Here's how the part is built. I have some questions about the finished solid (model axes, mm). A direction names the side the tool comes from. Coordinates: 2 decimals unless noted, no trailing zeros. Loops run counter-clockwise (first coordinate to the right, second up) from the corner with the lowest first, then second, coordinate; pieces in that order, holes last. Notation, with made-up numbers: (46.25, -16) - (99.25, -16) arc R16 cw to (99.25, -8) - close; hole circle Ø2 at (80.25, -29). An arc over 180 degrees is marked (long way). Use a Markdown table: item, result.
```python
from build123d import *

# Parameters (mm, degrees)
F1_DEPTH = 914.4
F2_W     = 762
F2_H     = 762
F3_DEPTH = 3.175
F4_R     = 12.7
F6_DEPTH = 228.6


with BuildPart() as f1:
    # F0 (on Top) → F1 (new body)
    with BuildSketch(Plane.XY):
        with BuildLine():
            Line((-19.3675, -30.95625), (0, -30.95625))
            Line((0, -30.95625), (19.3675, -30.95625))
            ThreePointArc((19.3675, -30.95625), (20.265526, -30.584276), (20.6375, -29.68625))
            Line((20.6375, -29.68625), (20.6375, 29.68625))
            ThreePointArc((20.6375, 29.68625), (20.265526, 30.584276), (19.3675, 30.95625))
            Line((19.3675, 30.95625), (15.5575, 30.95625))
            ThreePointArc((15.5575, 30.95625), (14.659474, 30.584276), (14.2875, 29.68625))
            Line((14.2875, 29.68625), (14.2875, 24.60625))
            Line((14.2875, 24.60625), (15.29505, 24.60625))
            Line((15.29505, 24.60625), (15.29505, 29.68625))
            ThreePointArc((15.29505, 29.68625), (15.37192, 29.87183), (15.5575, 29.9487))
            Line((15.5575, 29.9487), (19.3675, 29.9487))
            ThreePointArc((19.3675, 29.9487), (19.55308, 29.87183), (19.62995, 29.68625))
            Line((19.62995, 29.68625), (19.62995, -29.68625))
            ThreePointArc((19.62995, -29.68625), (19.55308, -29.87183), (19.3675, -29.9487))
            Line((19.3675, -29.9487), (0, -29.9487))
            Line((0, -29.9487), (-19.3675, -29.9487))
            ThreePointArc((-19.3675, -29.9487), (-19.55308, -29.87183), (-19.62995, -29.68625))
            Line((-19.62995, -29.68625), (-19.62995, 29.68625))
            ThreePointArc((-19.62995, 29.68625), (-19.55308, 29.87183), (-19.3675, 29.9487))
            Line((-19.3675, 29.9487), (-15.5575, 29.9487))
            ThreePointArc((-15.5575, 29.9487), (-15.37192, 29.87183), (-15.29505, 29.68625))
            Line((-15.29505, 29.68625), (-15.29505, 24.60625))
            Line((-15.29505, 24.60625), (-14.2875, 24.60625))
            Line((-14.2875, 24.60625), (-14.2875, 29.68625))
            ThreePointArc((-14.2875, 29.68625), (-14.659474, 30.584276), (-15.5575, 30.95625))
            Line((-15.5575, 30.95625), (-19.3675, 30.95625))
            ThreePointArc((-19.3675, 30.95625), (-20.265526, 30.584276), (-20.6375, 29.68625))
            Line((-20.6375, 29.68625), (-20.6375, -29.68625))
            ThreePointArc((-20.6375, -29.68625), (-20.265526, -30.584276), (-19.3675, -30.95625))
        make_face()
    extrude(amount=F1_DEPTH)

    # F2 (on Top) → F3 (join)
    with BuildSketch(Plane.XY):
        Rectangle(F2_W, F2_H)
    extrude(amount=-F3_DEPTH)

    # F4
    f4_edges = [f1.edges().sort_by_distance(p)[0] for p in [
        (381, -381, -1.5875),
        (381, 381, -1.5875),
        (-381, 381, -1.5875),
        (-381, -381, -1.5875),
    ]]
    fillet(f4_edges, radius=F4_R)

    # F5 (on Right) → F6 (join, symmetric)
    with BuildSketch(Plane.YZ):
        with BuildLine():
            Line((-29.9487, 915.67), (-29.9487, 954.405))
            ThreePointArc((-29.9487, 954.405), (-29.87183, 954.59058), (-29.68625, 954.66745))
            Line((-29.68625, 954.66745), (29.68625, 954.66745))
            ThreePointArc((29.68625, 954.66745), (29.87183, 954.59058), (29.9487, 954.405))
            Line((29.9487, 954.405), (29.9487, 950.595))
            ThreePointArc((29.9487, 950.595), (29.87183, 950.40942), (29.68625, 950.33255))
            Line((29.68625, 950.33255), (24.60625, 950.33255))
            Line((24.60625, 950.33255), (24.60625, 949.325))
            Line((24.60625, 949.325), (29.68625, 949.325))
            ThreePointArc((29.68625, 949.325), (30.584276, 949.696974), (30.95625, 950.595))
            Line((30.95625, 950.595), (30.95625, 954.405))
            ThreePointArc((30.95625, 954.405), (30.584276, 955.303026), (29.68625, 955.675))
            Line((29.68625, 955.675), (-29.68625, 955.675))
            ThreePointArc((-29.68625, 955.675), (-30.584276, 955.303026), (-30.95625, 954.405))
            Line((-30.95625, 954.405), (-30.95625, 935.0375))
            Line((-30.95625, 935.0375), (-30.95625, 915.67))
            ThreePointArc((-30.95625, 915.67), (-30.584276, 914.771974), (-29.68625, 914.4))
            Line((-29.68625, 914.4), (29.68625, 914.4))
            ThreePointArc((29.68625, 914.4), (30.584276, 914.771974), (30.95625, 915.67))
            Line((30.95625, 915.67), (30.95625, 919.48))
            ThreePointArc((30.95625, 919.48), (30.584276, 920.378026), (29.68625, 920.75))
            Line((29.68625, 920.75), (24.60625, 920.75))
            Line((24.60625, 920.75), (24.60625, 919.74245))
            Line((24.60625, 919.74245), (29.68625, 919.74245))
            ThreePointArc((29.68625, 919.74245), (29.87183, 919.66558), (29.9487, 919.48))
            Line((29.9487, 919.48), (29.9487, 915.67))
            ThreePointArc((29.9487, 915.67), (29.87183, 915.48442), (29.68625, 915.40755))
            Line((29.68625, 915.40755), (-29.68625, 915.40755))
            ThreePointArc((-29.68625, 915.40755), (-29.87183, 915.48442), (-29.9487, 915.67))
        make_face()
    extrude(amount=F6_DEPTH, both=True)


solid = f1.part
```
Q1. Will these pins go through, and if not, where does the flat tip stop? P1, Ø4, axis at x = -38, z = 953, coming from the +Y side; P2, Ø1.5, axis at x = -196.5, y = -188.5, coming from the +Z side; P3, Ø1.4, axis at x = -16.5, y = 30.5, coming from the +Z side.
Check values:
| item | result |
|---|---|
| P1 | y = 30.96 |
| P2 | z = 0 |
| P3 | z = 955.67 |
Q2. I want a section at C-C, the plane y = -71.5. Write out the boundary of the cut face in (x, z) (3 decimals).
Check values:
| item | result |
|---|---|
| outline | (-381, -3.175) - (381, -3.175) - (381, 0) - (-381, 0) - close |
Q3. Please list where these lines run through material, in increasing order: L1, parallel to Z at x = 170, y = -6.5 (3 decimals); L2, parallel to Z at x = 318, y = -3.5 (3 decimals). Write a range as from..to.
Check values:
| item | result |
|---|---|
| L1 | -3.175..0, 914.4..915.408, 954.667..955.675 |
| L2 | -3.175..0 |
Q4. Which directions (+Z, -Z, +X, -X, +Y, -Y) give clear straight access to the entire face, cutting with the end or side of a thin tool? Please do faces 1 (the face through (3, -30.956, 935)), 2 (the face through (-123, 0, 914.4)), 3 (the face through (20.638, 0, 451)), 4 (the face through (19.63, 0, 451)), 5 (the face through (3, 0, 954.667)).
Check values:
| item | result |
|---|---|
| face 1 | +Z, +X, -X, -Y |
| face 2 | -X, +Y, -Y |
| face 3 | +X, +Y, -Y |
| face 4 | none |
| face 5 | +X, -X |
Q5. If we mould it in two halves opening along X, with no side actions, what happens to faces 6 (the face through (228.6, -9, 915)), 7 (the face through (-19.63, 0, 451)), 8 (the face through (-5, 5, -3.175)), 9 (the face through (-20.638, 0, 451))? For each: pulls with the +X half, pulls with the -X half, needs draft (parallel to the pull), parting line crosses it, or undercut.
Check values:
| item | result |
|---|---|
| face 6 | pulls with the +X half |
| face 7 | undercut |
| face 8 | needs draft |
| face 9 | pulls with the -X half |
Q6. I want a section at B-B, the plane z = 859.5. Write out the boundary of the cut face in (x, y), then the cut area to 3 significant figures.
Check values:
| item | result |
|---|---|
| outline | (-20.64, -29.69) arc R1.27 ccw to (-19.37, -30.96) - (19.37, -30.96) arc R1.27 ccw to (20.64, -29.69) - (20.64, 29.69) arc R1.27 ccw to (19.37, 30.96) - (15.56, 30.96) arc R1.27 ccw to (14.29, 29.69) - (14.29, 24.61) - (15.3, 24.61) - (15.3, 29.69) arc R0.26 cw to (15.56, 29.95) - (19.37, 29.95) arc R0.26 cw to (19.63, 29.69) - (19.63, -29.69) arc R0.26 cw to (19.37, -29.95) - (-19.37, -29.95) arc R0.26 cw to (-19.63, -29.69) - (-19.63, 29.69) arc R0.26 cw to (-19.37, 29.95) - (-15.56, 29.95) arc R0.26 cw to (-15.3, 29.69) - (-15.3, 24.61) - (-14.29, 24.61) - (-14.29, 29.69) arc R1.27 ccw to (-15.56, 30.96) - (-19.37, 30.96) arc R1.27 ccw to (-20.64, 29.69) - close |
| area | 184 mm^2 |
